Autodesk Inventor part; units mm, degrees
ref_plane "YZ Plane" through (0, 0, 0) normal (1, 0, 0) x (0, 1, 0)
ref_plane "XZ Plane" through (0, 0, 0) normal (0, 1, 0) x (-1, 0, 0)
ref_plane "XY Plane" through (0, 0, 0) normal (0, 0, 1) x (1, 0, 0)
sketch "Sketch1" plane through (0, 0, 0) normal (0, 0, 1) x (1, 0, 0)
  line L0 (-41.275, -25.4) -> (41.275, -25.4)
  line L1 (41.275, -25.4) -> (41.275, 25.4)
  line L2 (41.275, 25.4) -> (-41.275, 25.4)
  line L3 (-41.275, 25.4) -> (-41.275, -25.4)
  line L4 (-41.275, -25.4) -> (41.275, 25.4) construction
  line L5 (41.275, -25.4) -> (-41.275, 25.4) construction
  point P0 (0, 0)
  dimension "d0" = 82.55
  dimension "d1" = 50.8
extrude "Extrusion1" add sketch "Sketch1" along normal blind 9.525
sketch "Sketch2" plane through (0, 0, 9.525) normal (0, 0, 1) x (1, 0, 0)
  line L0 (-28.575, -15.875) -> (28.575, -15.875)
  line L1 (-41.275, 25.4) -> (-41.275, -25.4)
  line L2 (-41.275, -25.4) -> (41.275, -25.4)
  point P0 (0, 0)
  dimension "d4" = 57.15
  dimension "d5" = 12.7
  dimension "d6" = 9.525
hole "Hole1" at (-28.575, -15.875, 9.525) at (28.575, -15.875, 9.525) direction (0, 0, -1) diameter 4.4958 depth 25.4 tip angle 118 counterbore diameter 7.9502 counterbore depth 2.54
sketch "Sketch3" plane through (0, 0, 9.525) normal (0, 0, 1) x (1, 0, 0)
  line L0 (-41.275, 25.4) -> (-41.275, -25.4)
  line L1 (-41.275, -25.4) -> (-41.275, 25.4)
  line L2 (-41.275, 25.4) -> (-52.275, 25.4)
  line L3 (-52.275, 25.4) -> (-52.275, -25.4)
  line L4 (-52.275, -25.4) -> (-41.275, -25.4)
  point P0 (0, 0)
  dimension "d14" = 11
extrude "Extrusion2" add sketch "Sketch3" against normal blind 4.953
sketch "Sketch4" plane through (0, 0, 4.572) normal (0, 0, -1) x (-1, 0, 0)
  line L0 (52.275, 25.4) -> (41.275, 25.4)
  line L1 (52.275, -25.4) -> (52.275, 25.4)
  point P0 (0, 0)
  point P1 (48.775, 11.43)
  dimension "d17" = 13.97
  dimension "d18" = 3.5
hole "Hole2" at (-48.775, 11.43, 4.572) direction (0, 0, 1) diameter 3.302 depth 12.2936 tip angle 118
sketch "Sketch5" plane through (-41.275, 25.4, 0) normal (0, 1, 0) x (1, 0, 0)
  line L0 (69.85, -6.35) -> (12.7, -6.35)
  line L1 (0, 0) -> (0, -4.572)
  line L2 (82.55, -9.525) -> (-11, -9.525)
  point P0 (41.275, 0)
  dimension "d26" = 57.15
  dimension "d27" = 12.7
  dimension "d28" = 3.175
hole "Hole3" at (-28.575, 25.4, 6.35) at (28.575, 25.4, 6.35) direction (0, -1, 0) diameter 2.6416 depth 10.9728 tip angle 118
properties part number "right side"
Source: CAD feature listing. Evaluate the final solid. Frame: model axes, mm. A direction names the side the tool comes from. Coordinates: 2 decimals unless noted, no trailing zeros. Loops run counter-clockwise (first coordinate to the right, second up) from the corner with the lowest first, then second, coordinate; pieces in that order, holes last. Notation, with made-up numbers: M 44,34.25 L 59,34.25 A6 ccw 59,39.25 Z; hole C 45.25,73 d11. An arc over 180 degrees is marked long. Answer in a Markdown table with one row per item.
Q1. Ray query, probe 1 along X at (y, z) = (17.75, 6.35) (3 decimals); probe 2 along X at (y, z) = (-13.5, 9) (3 decimals); probe 3 along X at (y, z) = (11.43, 7.3) (3 decimals). Return the intervals inside material, ascending. Write a range as from..to.
Answers below:
| item | result |
|---|---|
| probe 1 | x = -52.275..-29.896, -27.254..27.254, 29.896..41.275 |
| probe 2 | x = -52.275..-31.763, -25.387..25.387, 31.763..41.275 |
| probe 3 | x = -52.275..-50.426, -47.124..41.275 |
Q2. Set-up query: faces 4 (the flat face through (-47, 0, 4.572)), 5 (the cylindrical face through (32.456, -15.013, 8.237)), 6 (the cylindrical face through (29.379, 19.837, 5.302)), 7 (the flat face through (-5, 25.4, 5)). Return all of +Z, -Z, +X, -X, +Y, -Y with unobstructed straight access to the full face (end or side cutting, diameter ignored); none if empty.
Answers below:
| item | result |
|---|---|
| face 4 | -Z, -X, +Y, -Y |
| face 5 | +Z |
| face 6 | +Y |
| face 7 | +Z, -Z, +X, -X, +Y |
Q3. First-contact query: pin 1 (3.5 mm diameter, centred on y = -1.5, z = 2, fed in from -X) (3 decimals); pin 2 (4.5 mm diameter, centred on x = -48.775, y = 11.43, fed in from +Z) (3 decimals); pin 3 (2 mm diameter, centred on x = -28.575, z = 6.35, fed in from +Y); pin 4 (4 mm diameter, centred on x = -27.5, y = -15.5, fed in from +Z) (3 decimals). Flat tips, straight axial feed; report the tip coordinate or a pass-through.
Answers below:
| item | result |
|---|---|
| pin 1 | stops at x = -41.275 |
| pin 2 | stops at z = 9.525 |
| pin 3 | stops at y = 14.23 |
| pin 4 | stops at z = 6.985 |
Q4. Section B-B on z = 2.5. Return the cut outline in (x, y) (3 decimals).
Answers below:
| item | result |
|---|---|
| outline | M -41.275,-25.4 L 41.275,-25.4 L 41.275,25.4 L -41.275,25.4 Z; hole C -28.575,-15.875 d4.496; hole C 28.575,-15.875 d4.496 |
Q5. Draft query along Z for faces 1 (the flat face through (-41.275, 0, 2)), 2 (the flat face through (30, -18, 6.985)), 3 (the cylindrical face through (-29.885, 19.837, 6.178)). Return one class per face: pulls with the +Z half, pulls with the -Z half, needs draft (parallel to the pull), parting line crosses it, or undercut.
Answers below:
| item | result |
|---|---|
| face 1 | needs draft |
| face 2 | pulls with the +Z half |
| face 3 | undercut |
Q6. Section A-A on y = 11.43. Return the cut outline in (x, z) (3 decimals).
Answers below:
| item | result |
|---|---|
| outline | M -52.275,4.572 L -50.426,4.572 L -50.426,9.525 L -52.275,9.525 Z; M -47.124,4.572 L -41.275,4.572 L -41.275,0 L 41.275,0 L 41.275,9.525 L -47.124,9.525 Z |
Q7. Section C-C on y = -9. Return the cut outline in (x, z) (3 decimals).
Answers below:
| item | result |
|---|---|
| outline | M -52.275,4.572 L -41.275,4.572 L -41.275,0 L 41.275,0 L 41.275,9.525 L -52.275,9.525 Z |
